Geometry: final body of the model. Coordinates: model frame, mm. Round coordinates to 2 decimals unless told otherwise and drop trailing zeros. Loops run counter-clockwise (first coordinate to the right, second up) from the corner with the lowest first, then second, coordinate; pieces in that order, holes last. Notation, with made-up numbers: (65.25, -2.5) - (95.25, -2.5) arc R22 cw to (95.25, 10.5) - close; hole circle Ø4 at (-35, -20.5). An arc over 180 degrees is marked (long way). Answer as a JSON object with one key per item and string values. Group by question number.
Item 1: Section D-D (x = 16.75). Return the cut outline in (y, z).
Item 2: Section C-C (y = 4.75). Return the cut outline in (x, z).
Item 3: Line query: line 1 (Y direction, x = 17.75, z = 1.7); line 2 (Y direction, x = 14.25, z = 0.85); line 3 (Z direction, x = 15.25, y = 5.25). Output: solid intervals per line, ascending.
Item 4: Section A-A (x = 2.75). Return the cut outline in (y, z).
Item 5: First-contact query: pin 1 (1.7 mm diameter, centred on x = 2, y = 1, fed in from -Z); pin 2 (2.5 mm diameter, centred on x = 4.5, y = 1, fed in from +Z); pin 3 (1.5 mm diameter, centred on x = 7, z = 2, fed in from +Y). Flat tips, straight axial feed; report the tip coordinate or a pass-through.
Item 6: Section B-B (z = 2.65). Return the cut outline in (x, y).
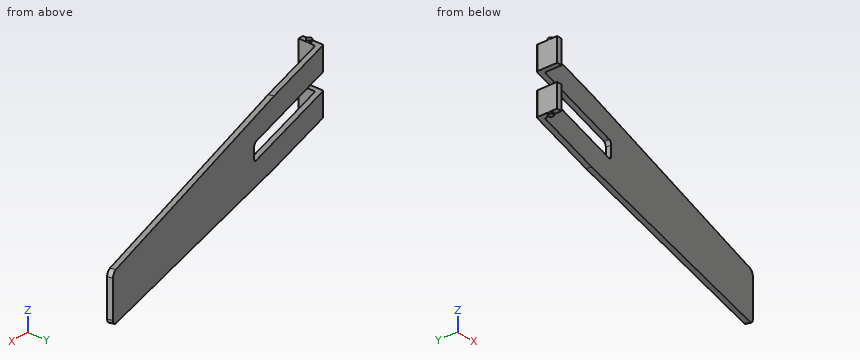
```python
from build123d import *

# Parameters (mm, degrees)
PROFILE_EXTRUDE_DEPTH   = 3.8
CHAMFER_TOP_SIZE        = 0.5
CHAMFER_TOP_SIZE2       = 16.846754467
PINS_EXTRUDE_DEPTH      = 0.1
PINS_EXTRUDE_DEPTH_BACK = 3.9
SKETCH3_R               = 0.15
SLOT_SKETCH_W           = 7
SLOT_SKETCH_H           = 1
SLOT_CUT_DEPTH          = 10
FILLET1_R               = 0.1
FILLET2_R               = 0.3
FILLET3_R               = 0.2


with BuildPart() as part:
    # Profile Sketch → Profile Extrude (new body)
    with BuildSketch(Plane.XY):
        Polygon((0, 0), (0, 1.230198096), (21.250368178, 6.924217089), (21.328013892, 6.634439341), (0.3, 1), (0.3, 0), align=None)
    extrude(amount=PROFILE_EXTRUDE_DEPTH)

    # Chamfer Top
    chamfer_top_edges = [part.edges().sort_by_distance(p)[0] for p in [
        (21.289191035, 6.779328215, 3.8),
        (21.289191035, 6.779328215, 0),
    ]]
    chamfer_top_side = [part.faces().sort_by_distance(p)[0] for p in [
        (21.289191035, 6.779328215, 1.9),
    ]]
    chamfer(chamfer_top_edges, length=CHAMFER_TOP_SIZE, length2=CHAMFER_TOP_SIZE2, reference=chamfer_top_side[0])

    # Sketch3 → Pins Extrude (add, two sides: drawn at the far end of the back side and taken through both)
    with BuildSketch(Plane.XY.offset(3.8).offset(-PINS_EXTRUDE_DEPTH_BACK)):
        with Locations((0.15, 0.5)):
            Circle(SKETCH3_R)
    extrude(amount=PINS_EXTRUDE_DEPTH + PINS_EXTRUDE_DEPTH_BACK)

    # Slot Sketch → Slot Cut (cut)
    with BuildSketch(Plane.XZ):
        with Locations((3.5, 1.9)):
            Rectangle(SLOT_SKETCH_W, SLOT_SKETCH_H)
    extrude(amount=-SLOT_CUT_DEPTH, mode=Mode.SUBTRACT)

    # Fillet1
    fillet1_edges = [part.edges().sort_by_distance(p)[0] for p in [
        (0, 1.230198096, 3.1),
        (0.3, 1, 3.1),
        (0, 1.230198096, 0.7),
        (0.3, 1, 0.7),
    ]]
    fillet(fillet1_edges, radius=FILLET1_R)

    # Fillet2
    fillet2_edges = [part.edges().sort_by_distance(p)[0] for p in [
        (21.289191035, 6.779328215, 0.5),
        (21.289191035, 6.779328215, 3.3),
    ]]
    fillet(fillet2_edges, radius=FILLET2_R)

    # Fillet3
    fillet3_edges = [part.edges().sort_by_distance(p)[0] for p in [
        (7, 2.950551016, 2.4),
        (7, 2.950551016, 1.4),
    ]]
    fillet(fillet3_edges, radius=FILLET3_R)


solid = part.part
```
Values:
{
 "1": {"outline": "(5.41, 0.36) - (5.72, 0.36) - (5.72, 3.44) - (5.41, 3.44) - close"},
 "2": {"outline": "(13.14, 0.25) - (14.3, 0.28) - (14.3, 3.52) - (13.14, 3.55) - close"},
 "3": {"line 1": "y = 5.68 to 5.99", "line 2": "y = 4.74 to 5.05", "line 3": "z = 0.32 to 3.48"},
 "4": {"outline": "(1.66, 0) - (1.97, 0) - (1.97, 1.4) - (1.66, 1.4) - close; (1.66, 2.4) - (1.97, 2.4) - (1.97, 3.8) - (1.66, 3.8) - close"},
 "5": {"pin 1": "stops at z = 0", "pin 2": "stops at z = 3.8", "pin 3": "stops at y = 3.31"},
 "6": {"outline": "(0, 0) - (0.3, 0) - (0.3, 0.92) arc R0.1 cw to (0.37, 1.02) - (21.33, 6.63) - (21.25, 6.92) - (0.07, 1.25) arc R0.1 ccw to (0, 1.15) - close"}
}
